from build123d import *

# Parameters (mm, degrees)
F1_DEPTH  = 254
F2_R      = 381
F3_DEPTH  = 355.6
F4_R      = 76.2
F5_DEPTH  = 254
F6_R      = 76.2
F7_DEPTH  = 254
F8_R      = 114.3
F8_R_2    = 76.2
F9_DEPTH  = 127
F10_DEPTH = 25.4
F11_R     = 114.3
F12_DEPTH = 127
F13_R     = 254
F14_DEPTH = 609.6
F15_R     = 304.8
F16_DEPTH = 101.6


with BuildPart() as f1:
    # F0 (on Top) → F1 (new body)
    with BuildSketch(Plane.XY):
        with BuildLine():
            ThreePointArc((87.085714, -370.913842), (298.614013, -236.62348), (381, 0))
            ThreePointArc((381, 0), (298.614013, 236.62348), (87.085714, 370.913842))
            ThreePointArc((87.085714, 370.913842), (0, 381), (-87.085714, 370.913842))
            ThreePointArc((-87.085714, 370.913842), (-381, 0), (-87.085714, -370.913842))
            ThreePointArc((-87.085714, -370.913842), (0, -381), (87.085714, -370.913842))
        make_face()
        with BuildLine():
            ThreePointArc((87.085714, 370.913842), (298.614013, 236.62348), (381, 0))
            ThreePointArc((381, 0), (298.614013, -236.62348), (87.085714, -370.913842))
            Line((87.085714, -370.913842), (929.64, -173.093126))
            ThreePointArc((929.64, -173.093126), (1066.8, 0), (929.64, 173.093126))
            Line((929.64, 173.093126), (87.085714, 370.913842))
        make_face()
        with BuildLine():
            ThreePointArc((-87.085714, -370.913842), (-381, 0), (-87.085714, 370.913842))
            Line((-87.085714, 370.913842), (-929.64, 173.093126))
            ThreePointArc((-929.64, 173.093126), (-1066.8, 0), (-929.64, -173.093126))
            Line((-929.64, -173.093126), (-87.085714, -370.913842))
        make_face()
    extrude(amount=-F1_DEPTH)

    # F2 (on face) → F3 (join)
    with BuildSketch(Plane.XY):
        Circle(F2_R)
    extrude(amount=F3_DEPTH)

    # F4 (on face) → F5 (cut)
    with BuildSketch(Plane.XY):
        with Locations((-889, 0)):
            Circle(F4_R)
    extrude(amount=-F5_DEPTH, mode=Mode.SUBTRACT)

    # F6 (on face) → F7 (cut)
    with BuildSketch(Plane.XY):
        with Locations((889, 0)):
            Circle(F6_R)
    extrude(amount=-F7_DEPTH, mode=Mode.SUBTRACT)

    # F8 (on face) → F9 (cut)
    with BuildSketch(Plane.XY):
        with Locations((-889, 0)):
            Circle(F8_R)
        with Locations((-889, 0)):
            Circle(F8_R_2, mode=Mode.SUBTRACT)
    extrude(amount=-F9_DEPTH, mode=Mode.SUBTRACT)

    # F8 (on face) → F10 (cut)
    with BuildSketch(Plane.XY):
        with Locations((-889, 0)):
            Circle(F8_R)
        with Locations((-889, 0)):
            Circle(F8_R_2, mode=Mode.SUBTRACT)
    extrude(amount=-F10_DEPTH, mode=Mode.SUBTRACT)

    # F11 (on face) → F12 (cut)
    with BuildSketch(Plane.XY):
        with Locations((889, 0)):
            Circle(F11_R)
    extrude(amount=-F12_DEPTH, mode=Mode.SUBTRACT)

    # F13 (on face) → F14 (cut)
    with BuildSketch(Plane.XY.offset(355.6)):
        Circle(F13_R)
    extrude(amount=-F14_DEPTH, mode=Mode.SUBTRACT)

    # F15 (on face) → F16 (cut)
    with BuildSketch(Plane.XY.offset(355.6)):
        Circle(F15_R)
    extrude(amount=-F16_DEPTH, mode=Mode.SUBTRACT)


solid = f1.part
CAD build for the part. Positions are in the model's coordinates, mm. A direction names the side the tool comes from. Give positions to 0.01 mm unless a question says otherwise; leave off trailing zeros. Loops run counter-clockwise (first coordinate to the right, second up) from the corner with the lowest first, then second, coordinate; pieces in that order, holes last. Notation, with made-up numbers: M -6,12 L 40,12 A8 cw 40,20 Z; hole C 18.5,-11.5 d11. An arc over 180 degrees is marked long. One line per question, with ' | ' between items. Start each with the question number.
1. Saw through at D-D on y = 141.5. Give the cut face in (x, z), plus the area to 3 significant figures.
2. Two-plate mould, pull along Y, no slides. Class faces 1 (the face through (-514.26, -270.62, -125.22)), 2 (the face through (998.022, 34.333, -62.611)), 3 (the face through (1066.77, -3.34, -125.22)): pulls with the +Y half, pulls with the -Y half, needs draft (parallel to the pull), parting line crosses it, or undercut.
3. Saw through at A-A on y = 0. State how many separate pieces and enclosed holes the cut face has, plus the area to 3 significant figures.
4. Probe L1, parallel to Y at x = 0, z = 324; L2, parallel to X at y = 98, z = -64; L3, parallel to X at y = -48, z = -103. List the from-to ranges inside material, lowest first. Write a range as from..to.
5. Flat gauge pins, fed straight in: pin 1 (1 mm diameter, centred on y = 30.5, z = -179.5, fed in from +X); pin 2 (2 mm diameter, centred on x = -87.5, z = 273, fed in from +Y); pin 3 (3 mm diameter, centred on x = 242.5, z = -140.5, fed in from +Y). Where does each tip first touch, or does it go through?
6. Saw through at B-B on z = -80. Give the cut face in (x, y), plus the area to 3 significant figures.
7. Saw through at C-C on x = 889. Give the cut face in (y, z), plus the area to 3 significant figures.
8. 3-axis set-ups, long thin cutter, end or side, ignore diameter. For faces 4 (the face through (-502.46, 273.39, -125.22)), 5 (the face through (-302.35, -231.83, 175.31)): which of +Z, -Z, +X, -X, +Y, -Y reach the whole face in a straight line?
Result sheet:
1) outline: M -996.66,-254 L -210.94,-254 L -210.94,254 L -269.96,254 L -269.96,355.6 L -353.75,355.6 L -353.75,0 L -996.66,0 Z; M 210.94,-254 L 996.66,-254 L 996.66,0 L 353.75,0 L 353.75,355.6 L 269.96,355.6 L 269.96,254 L 210.94,254 Z | area: 489,000 mm^2
2) face 1: pulls with the -Y half | face 2: undercut | face 3: parting line crosses it
3) separate pieces: 4 | enclosed holes: 0 | area: 396,000 mm^2
4) L1: y = -381..-304.8, 304.8..381 | L2: x = -1037.35..-947.83, -830.17..-234.33, 234.33..830.17, 947.83..1037.35 | L3: x = -1060.2..-992.73, -785.27..-249.42, 249.42..785.27, 992.73..1060.2
5) pin 1: stops at x = 1064.25 | pin 2: stops at y = 371.05 | pin 3: stops at y = 334.78
6) outline: M -929.64,-173.09 L -87.09,-370.91 A381 ccw 87.09,-370.91 L 929.64,-173.09 A177.8 ccw 929.64,173.09 L 87.09,370.91 A381 ccw -87.09,370.91 L -929.64,173.09 A177.8 ccw Z; hole C -889,0 d228.6; hole C 0,0 d508; hole C 889,0 d228.6 | area: 834,000 mm^2
7) outline: M -182.63,-254 L -76.2,-254 L -76.2,-127 L -114.3,-127 L -114.3,0 L -182.63,0 Z; M 76.2,-254 L 182.63,-254 L 182.63,0 L 114.3,0 L 114.3,-127 L 76.2,-127 Z | area: 44,400 mm^2
8) face 4: +Z, -Z, -X, +Y | face 5: +Z
